Here's how the part is built. I have some questions about the finished solid (model axes, mm). A direction names the side the tool comes from. Round coordinates to 2 decimals unless told otherwise and drop trailing zeros. Loops run counter-clockwise (first coordinate to the right, second up) from the corner with the lowest first, then second, coordinate; pieces in that order, holes last. Notation, with made-up numbers: (-12.75, -7.75) - (-6.75, -7.75) arc R14 ccw to (-6.75, 5.25) - close; hole circle Ø5 at (0, 71.25). An arc over 180 degrees is marked (long way). Return JSON: item names as keys, results as strings. Group by question number.
```python
from build123d import *

# Parameters (mm, degrees)
SM_BASE_FLANGE_1_DEPTH             = 8
SM_EDGE_FLANGE_1_STRIP_W           = 48
SM_EDGE_FLANGE_1_STRIP_H           = 8
SM_EDGE_FLANGE_1_STRIP_CUT_DEPTH   = 2325
SM_EDGE_FLANGE_1_STRIP_2_W         = 48
SM_EDGE_FLANGE_1_STRIP_2_H         = 8
SM_EDGE_FLANGE_1_STRIP_CUT_2_DEPTH = 2295
SM_EDGE_FLANGE_1_RELIEF_W          = 52
SM_EDGE_FLANGE_1_RELIEF_H          = 4
SM_EDGE_FLANGE_1_RELIEF_CUT_DEPTH  = 8
SM_EDGE_FLANGE_1_DEPTH             = 2325
SM_EDGE_FLANGE_1_BEND_DEPTH        = 2295
CHAMFER_1_SIZE                     = 4
SKETCH_12_R                        = 45
CUT_EXTRUDE_1_DEPTH                = 2337.029537484


# Sheet-metal steps are written as plain solids
with BuildPart() as part:
    # Sketch 1 → 基体-法兰1 (new body)
    with BuildSketch(Plane(origin=(0, 0, 0), x_dir=(0, 0, -1), z_dir=(1, 0, 0))):
        Polygon((0, 0), (2325, 0), (2325, -215), (30, -215), (0, -185), align=None)
    extrude(amount=-SM_BASE_FLANGE_1_DEPTH)

    # 边线-法兰1 strip (across the edge) → 边线-法兰1 strip cut (cut)
    with BuildSketch(Plane(origin=(0, 0, -2325), x_dir=(0, -1, 0), z_dir=(0, 0, 1))):
        with Locations((-8, -4)):
            Rectangle(SM_EDGE_FLANGE_1_STRIP_W, SM_EDGE_FLANGE_1_STRIP_H)
    extrude(amount=SM_EDGE_FLANGE_1_STRIP_CUT_DEPTH, mode=Mode.SUBTRACT)

    # 边线-法兰1 strip 2 (across the edge) → 边线-法兰1 strip cut 2 (cut)
    with BuildSketch(Plane(origin=(0, -215, -30), x_dir=(0, 1, 0), z_dir=(0, 0, -1))):
        with Locations((-8, -4)):
            Rectangle(SM_EDGE_FLANGE_1_STRIP_2_W, SM_EDGE_FLANGE_1_STRIP_2_H)
    extrude(amount=SM_EDGE_FLANGE_1_STRIP_CUT_2_DEPTH, mode=Mode.SUBTRACT)

    # 边线-法兰1 relief (on the sheet) → 边线-法兰1 relief cut (cut)
    with BuildSketch(Plane(origin=(0, -199, -30), x_dir=(0, 1, 0), z_dir=(1, 0, 0))):
        with Locations((-22, 2)):
            Rectangle(SM_EDGE_FLANGE_1_RELIEF_W, SM_EDGE_FLANGE_1_RELIEF_H)
    extrude(amount=-SM_EDGE_FLANGE_1_RELIEF_CUT_DEPTH, mode=Mode.SUBTRACT)

    # 边线-法兰1 section (across the edge) → 边线-法兰1 (add)
    with BuildSketch(Plane(origin=(0, 0, -2325), x_dir=(0, -1, 0), z_dir=(0, 0, 1))):
        with BuildLine():
            Line((0, 8), (0, 72))
            Line((0, 72), (8, 72))
            Line((8, 72), (8, 8))
            ThreePointArc((8, 8), (10.343145751, 2.343145751), (16, 0))
            Line((16, 0), (16, -8))
            ThreePointArc((16, -8), (4.686291501, -3.313708499), (0, 8))
        make_face()
    extrude(amount=SM_EDGE_FLANGE_1_DEPTH)

    # 边线-法兰1 section 2 (across the edge) → 边线-法兰1 bend (add)
    with BuildSketch(Plane(origin=(0, -215, -30), x_dir=(0, 1, 0), z_dir=(0, 0, -1))):
        with BuildLine():
            Line((0, 8), (0, 72))
            Line((0, 72), (8, 72))
            Line((8, 72), (8, 8))
            ThreePointArc((8, 8), (10.343145751, 2.343145751), (16, 0))
            Line((16, 0), (16, -8))
            ThreePointArc((16, -8), (4.686291501, -3.313708499), (0, 8))
        make_face()
    extrude(amount=SM_EDGE_FLANGE_1_BEND_DEPTH)

    # 倒角1
    chamfer_1_edges = [part.edges().sort_by_distance(p)[0] for p in [
        (72, 0, -1162.5),
        (72, -215, -1177.5),
    ]]
    chamfer(chamfer_1_edges, length=CHAMFER_1_SIZE)

    # 草图12 → 切除-拉伸1 (cut, through all)
    with BuildSketch(Plane(origin=(0, 0, 0), x_dir=(0, 0, -1), z_dir=(1, 0, 0))):
        with Locations((620, -107.5)):
            Circle(SKETCH_12_R)
    extrude(amount=-CUT_EXTRUDE_1_DEPTH, mode=Mode.SUBTRACT)


solid = part.part
```
Q1. Please list where these lines run through material, in increasing order: line 1 (Y direction, x = -6, z = -620); line 2 (Y direction, x = 36, z = -1228); line 3 (Z direction, x = -5, y = -107).
Q2. If we mould it in two halves opening along Y, with no side actions, what happens to faces 3 (the flat face through (38, 0, -1179)), 4 (the flat face through (40, -8, -1179)), 5 (the flat face through (-0.4, -115, -2325))? For each: +Y half, -Y half, draft (parallel to the pull), parting line (faces both ways), or undercut.
Q3. Imagine slicing it at C-C, the plane y = -107.5. List the corners of the cut face in (x, z) for me.
Q4. Imagine slicing it at D-D, the plane z = -1741. List the corners of the cut face in (x, y) for me.
Q5. Imagine slicing it at A-A, the plane x = 26.5. List the corners of the cut face in (y, z) for me.
Q6. Imagine slicing it at B-B, the plane z = -620. List the corners of the cut face in (x, y) for me.
Q7. For faces 1 (the flat face through (-8, -112, -1179)), 2 (the flat face through (0, -112, -1179)), which set-ups out of +Z, -Z, +X, -X, +Y, -Y let a thin tool reach every point of the face, with its end or its side?
Q8. Will these pins go through, and if not, where does the flat tip stop? pin 1 Ø3 at (y, z) = (-35.5, -259.5) entering from +X; pin 2 Ø1.2 at (x, z) = (-4, -27.5) entering from -Y; pin 3 Ø22 at (x, y) = (33.5, -200) entering from +Z.
Output values:
{
 "1": {"line 1": "y = -206.75 to -152.5, -62.5 to -8.25", "line 2": "y = -215 to -207, -8 to 0", "line 3": "z = -2325 to -665, -575 to 0"},
 "2": {"face 3": "+Y half", "face 4": "undercut", "face 5": "draft"},
 "3": {"outline": "(-8, -2325) - (0, -2325) - (0, -665) - (-8, -665) - close; (-8, -575) - (0, -575) - (0, 0) - (-8, 0) - close"},
 "4": {"outline": "(-8, -199) arc R16 ccw to (8, -215) - (68, -215) - (72, -211) - (72, -207) - (8, -207) arc R8 cw to (0, -199) - (0, -16) arc R8 cw to (8, -8) - (72, -8) - (72, -4) - (68, 0) - (8, 0) arc R16 ccw to (-8, -16) - close"},
 "5": {"outline": "(-215, -2325) - (-207, -2325) - (-207, -30) - (-215, -30) - close; (-8, -2325) - (0, -2325) - (0, 0) - (-8, 0) - close"},
 "6": {"outline": "(-8, -199) arc R16 ccw to (8, -215) - (68, -215) - (72, -211) - (72, -207) - (8, -207) arc R8 cw to (0, -199) - (0, -152.5) - (-8, -152.5) - close; (-8, -62.5) - (0, -62.5) - (0, -16) arc R8 cw to (8, -8) - (72, -8) - (72, -4) - (68, 0) - (8, 0) arc R16 ccw to (-8, -16) - close"},
 "7": {"face 1": "+Z, -Z, -X, +Y, -Y", "face 2": "+Z, -Z, +X"},
 "8": {"pin 1": "stops at x = 0", "pin 2": "stops at y = -195", "pin 3": "stops at z = -30"}
}
